```python
from build123d import *

# Parameters (mm, degrees)
SKETCH1_R           = 50
SKETCH1_W           = 20
SKETCH1_H           = 20
BOSS_EXTRUDE1_DEPTH = 20
SKETCH1_2_W         = 20
SKETCH1_2_H         = 20
BOSS_EXTRUDE2_DEPTH = 240


with BuildPart() as part:
    # Sketch1 → Boss-Extrude1 (new body)
    with BuildSketch(Plane(origin=(0, 0, 0), x_dir=(1, 0, 0), z_dir=(0, 1, 0))):
        Circle(SKETCH1_R)
        Rectangle(SKETCH1_W, SKETCH1_H, mode=Mode.SUBTRACT)
    extrude(amount=BOSS_EXTRUDE1_DEPTH)

    # Sketch1<2> → Boss-Extrude2 (add)
    with BuildSketch(Plane(origin=(0, 0, 0), x_dir=(1, 0, 0), z_dir=(0, 1, 0))):
        Rectangle(SKETCH1_2_W, SKETCH1_2_H)
    extrude(amount=BOSS_EXTRUDE2_DEPTH)


solid = part.part
```
Here's how the part is built. I have some questions about the finished solid (model axes, mm). A direction names the side the tool comes from. Round coordinates to 2 decimals unless told otherwise and drop trailing zeros. Write each loop counter-clockwise with the first axis right and the second up, starting at its lowest first coordinate (ties: lowest second). Pieces come first, ordered by that corner, then holes.
Q1. Which directions (+Z, -Z, +X, -X, +Y, -Y) give clear straight access to the entire face, cutting with the end or side of a thin tool? Please do faces 1 (the flat face through (0, 128, 10)), 2 (the flat face through (0, 128, -10)), 3 (the flat face through (-1, 0, -1)), 4 (the flat face through (10, 128, 0)), 5 (the flat face through (-10, 128, 0)).
Q2. If we section it at C-C on y = 107.5: Write out the boundary of the cut face in (x, z).
Q3. Please list where these lines run through material, in increasing order: probe 1 along Y at (x, z) = (-29, 22.5); probe 2 along X at (y, z) = (169, -3).
Q4. If we section it at A-A on x = 0: Write out the boundary of the cut face in (y, z).
Q5. If we section it at B-B on z = 0: Write out the boundary of the cut face in (x, y).
Q6. Will these pins go through, and if not, where does the flat tip stop? P1, Ø6, axis at x = 2.5, y = 141.5, coming from the -Z side; P2, Ø10, axis at x = -2.5, y = 147.5, coming from the +Z side; P3, Ø6, axis at y = 177, z = 4, coming from the +X side.
Q7. If we section it at D-D on x = 16: Write out the boundary of the cut face in (y, z).
Answer below:
1. face 1: +Z, +X, -X, +Y
1. face 2: -Z, +X, -X, +Y
1. face 3: +Z, -Z, +X, -X, -Y
1. face 4: +Z, -Z, +X, +Y
1. face 5: +Z, -Z, -X, +Y
2. outline: (-10, -10) - (10, -10) - (10, 10) - (-10, 10) - close
3. probe 1: y = 0 to 20
3. probe 2: x = -10 to 10
4. outline: (0, -50) - (20, -50) - (20, -10) - (240, -10) - (240, 10) - (20, 10) - (20, 50) - (0, 50) - close
5. outline: (-50, 0) - (50, 0) - (50, 20) - (10, 20) - (10, 240) - (-10, 240) - (-10, 20) - (-50, 20) - close
6. P1: stops at z = -10
6. P2: stops at z = 10
6. P3: stops at x = 10
7. outline: (0, -47.37) - (20, -47.37) - (20, 47.37) - (0, 47.37) - close
